```python
from build123d import *

# Parameters (mm, degrees)
PAD002_DEPTH  = 33
SKETCH003_W   = 165.06
SKETCH003_H   = 80.96
SKETCH003_W_2 = 23.5
SKETCH003_H_2 = 44.52
PAD003_DEPTH  = 10
SKETCH004_R   = 31
SKETCH004_R_2 = 29.055
PAD004_DEPTH  = 3
SKETCH033_W   = 165.06
SKETCH033_H   = 10
SKETCH033_H_2 = 15
PAD029_DEPTH  = 24.4
SKETCH034_W   = 23.5
SKETCH034_H   = 6
SKETCH034_R   = 1.15
PAD030_DEPTH  = 0.65


with BuildPart() as part:
    # Sketch002 → Pad002 (new body)
    with BuildSketch(Plane.XY):
        with BuildLine():
            ThreePointArc((-22.083648, 12.75), (0, -25.5), (22.083648, 12.75))
            ThreePointArc((-22.083648, 12.75), (0, -28.556543), (22.083648, 12.75))
        make_face()
    extrude(amount=PAD002_DEPTH)

    # Sketch003 → Pad003 (join)
    with BuildSketch(Plane.XY):
        with Locations((0, -11.48)):
            Rectangle(SKETCH003_W, SKETCH003_H)
        with BuildLine():
            ThreePointArc((-6.689544, 7.7), (-10.2, 0), (-6.689544, -7.7))
            Line((-6.689544, -7.7), (6.689544, -7.7))
            ThreePointArc((6.689544, -7.7), (10.2, 0), (6.689544, 7.7))
            Line((-6.689544, 7.7), (6.689544, 7.7))
        make_face(mode=Mode.SUBTRACT)
        with Locations((45, -4.35)):
            Rectangle(SKETCH003_W_2, SKETCH003_H_2, mode=Mode.SUBTRACT)
        with Locations((-45, -4.35)):
            Rectangle(SKETCH003_W_2, SKETCH003_H_2, mode=Mode.SUBTRACT)
    extrude(amount=-PAD003_DEPTH)

    # Sketch004 (on Face3 of Pad003) → Pad004 (join)
    with BuildSketch(Plane.XY):
        with Locations((0, -2)):
            Circle(SKETCH004_R)
        with Locations((0, -2)):
            Circle(SKETCH004_R_2, mode=Mode.SUBTRACT)
    extrude(amount=PAD004_DEPTH)

    # Sketch033 (on Face11 of Pad004) → Pad029 (join)
    with BuildSketch(Plane(origin=(0, 0, -10), x_dir=(1, 0, 0), z_dir=(0, 0, -1))):
        with Locations((0, -24)):
            Rectangle(SKETCH033_W, SKETCH033_H)
        with Locations((0, 44.46)):
            Rectangle(SKETCH033_W, SKETCH033_H_2)
    extrude(amount=PAD029_DEPTH)

    # Sketch034 (on Face25 of Pad029) → Pad030 (join)
    with BuildSketch(Plane.XY):
        with Locations((45, 14.91)):
            Rectangle(SKETCH034_W, SKETCH034_H)
        with Locations((35.9, 15.75)):
            Circle(SKETCH034_R, mode=Mode.SUBTRACT)
        with Locations((54.1, 15.75)):
            Circle(SKETCH034_R, mode=Mode.SUBTRACT)
        with Locations((45, -23.61)):
            Rectangle(SKETCH034_W, SKETCH034_H)
        with Locations((35.9, -24.45)):
            Circle(SKETCH034_R, mode=Mode.SUBTRACT)
        with Locations((54.1, -24.45)):
            Circle(SKETCH034_R, mode=Mode.SUBTRACT)
        with Locations((-45, 14.91)):
            Rectangle(SKETCH034_W, SKETCH034_H)
        with Locations((-35.9, 15.75)):
            Circle(SKETCH034_R, mode=Mode.SUBTRACT)
        with Locations((-54.1, 15.75)):
            Circle(SKETCH034_R, mode=Mode.SUBTRACT)
        with Locations((-45, -23.61)):
            Rectangle(SKETCH034_W, SKETCH034_H)
        with Locations((-35.9, -24.45)):
            Circle(SKETCH034_R, mode=Mode.SUBTRACT)
        with Locations((-54.1, -24.45)):
            Circle(SKETCH034_R, mode=Mode.SUBTRACT)
    extrude(amount=-PAD030_DEPTH)


solid = part.part
```
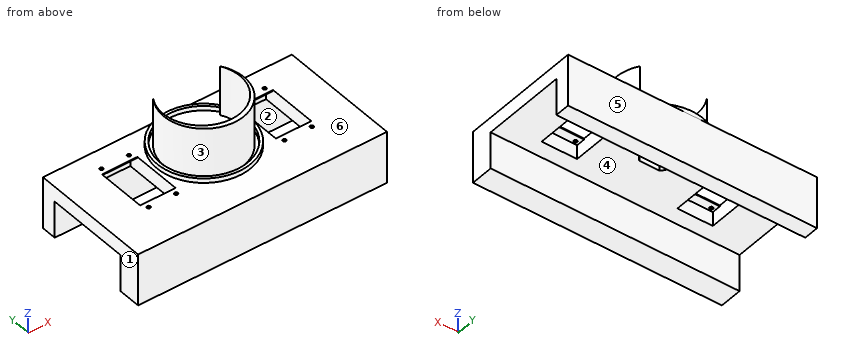
Can you work these out from the model? Positions are in its coordinate system, mm. Face numbers are marked on the shaded views. A direction names the side the tool comes from. Round coordinates to 2 decimals unless told otherwise and drop trailing zeros. Loops run counter-clockwise (first coordinate to the right, second up) from the corner with the lowest first, then second, coordinate; pieces in that order, holes last. Notation, with made-up numbers: M -24,53.5 L -20,53.5 A26 ccw -20,69.5 Z; hole C 88,13 d9. An arc over 180 degrees is marked long. Answer as a JSON object with one key per item and string values. Group by question number.
Q1. Imagine slicing it at A-A, the plane z = -21.5. Please give me the cut outline in (x, y), then the cut area to 3 significant figures.
Q2. Will these pins go through, and if not, where does the flat tip stop? pin 1 (4 mm diameter, centred on y = 1, z = 25.5, fed in from -X); pin 2 (12 mm diameter, centred on x = -31, y = 9, fed in from +Z); pin 3 (12 mm diameter, centred on x = 54.5, y = -28, fed in from -Z).
Q3. Imagine slicing it at D-D, the plane z = -4.5. Please give me the cut outline in (x, y).
Q4. Imagine slicing it at B-B, the plane x = -65. Please give me the cut outline in (y, z).
Q5. We'd pull the mould along Y, two halves only. Please class the marked faces 4, 5 and 6: +Y half, -Y half, draft (parallel to the pull), parting line (faces both ways), or undercut.
Q6. On a 3-axis mill with a long thin cutter (end or side, diameter ignored), from which of +Z, -Z, +X, -X, +Y, -Y can I reach the whole of each face in a straight line? I mean the marked faces 1, 2 and 3. Say none if no direction works.
Q7. Imagine slicing it at C-C, the plane y = -5. Count the separate pieces of the cut face and the enclosed holes in it, then the cut area to 3 significant figures.
Q8. Please list where these lines run through material, in increasing order: L1, parallel to Y at x = -35.9, z = -0.2; L2, parallel to Y at x = 61, z = -29.5; L3, parallel to X at y = 4, z = -3.
Findings:
{
 "1": {"outline": "M -82.53,-51.96 L 82.53,-51.96 L 82.53,-36.96 L -82.53,-36.96 Z; M -82.53,19 L 82.53,19 L 82.53,29 L -82.53,29 Z", "area": "4,130 mm2"},
 "2": {"pin 1": "stops at x = -26.54", "pin 2": "stops at z = 3", "pin 3": "stops at z = -10"},
 "3": {"outline": "M -82.53,-51.96 L 82.53,-51.96 L 82.53,29 L -82.53,29 Z; hole M -56.75,-26.61 L -33.25,-26.61 L -33.25,17.91 L -56.75,17.91 Z; hole M -6.69,-7.7 L 6.69,-7.7 A10.2 ccw 6.69,7.7 L -6.69,7.7 A10.2 ccw Z; hole M 33.25,-26.61 L 56.75,-26.61 L 56.75,17.91 L 33.25,17.91 Z"},
 "4": {"outline": "M -51.96,-34.4 L -36.96,-34.4 L -36.96,-10 L 19,-10 L 19,-34.4 L 29,-34.4 L 29,0 L -51.96,0 Z"},
 "5": {"face 4": "undercut", "face 5": "+Y half", "face 6": "draft"},
 "6": {"face 1": "+Z, -Z, -X, +Y, -Y", "face 2": "-Z, +X, -X", "face 3": "+Z"},
 "7": {"separate pieces": "4", "enclosed holes": "0", "area": "1,110 mm2"},
 "8": {"L1": "y = -51.96 to -25.6, -23.3 to -20.61, 11.91 to 14.6, 16.9 to 29", "L2": "y = -51.96 to -36.96, 19 to 29", "L3": "x = -82.53 to -56.75, -33.25 to -9.38, 9.38 to 33.25, 56.75 to 82.53"}
}
